```python
from build123d import *

# Parameters (mm, degrees)
SKETCH_2_R          = 0.8
CUT_EXTRUDE_1_DEPTH = 10
CHAMFER_1_SIZE      = 0.5


with BuildPart() as part:
    # Эскиз1 → Повернуть1 (revolve)
    with BuildSketch(Plane(origin=(0, 0, 0), x_dir=(0, 0, -1), z_dir=(1, 0, 0))):
        Polygon((0, 2.5), (0, 5), (2, 5), (2, 3), (38, 3), (38, 2.5), (42, 2.5), (42, 2.95), (43, 2.95), (43, 0), (0, 0), (-5, 0), (-5, 2.95), (-4, 2.95), (-4, 2.5), align=None)
    revolve(axis=Axis((0, 0, 0), (0, 0, -1)))

    # Эскиз2 → Вытянуть1 (cut, symmetric)
    with BuildSketch(Plane(origin=(0, 0, 0), x_dir=(0, 0, -1), z_dir=(1, 0, 0))):
        with Locations((36, 0)):
            Circle(SKETCH_2_R)
    extrude(amount=CUT_EXTRUDE_1_DEPTH, both=True, mode=Mode.SUBTRACT)

    # Фаска1
    chamfer_1_edges = [part.edges().sort_by_distance(p)[0] for p in [
        (0, -2.95, -43),
        (0, -2.95, 5),
    ]]
    chamfer(chamfer_1_edges, length=CHAMFER_1_SIZE)


solid = part.part
```
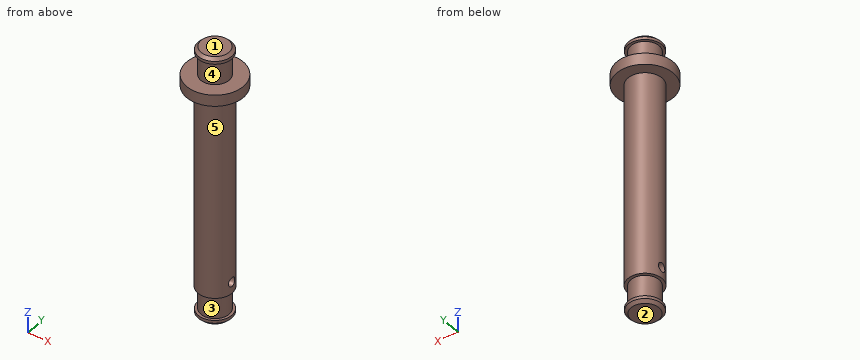
The listing builds one solid part. Answer for the finished solid, in the listing's coordinates (mm). Face numbers are marked on the shaded views. A direction names the side the tool comes from. Coordinates: 2 decimals unless noted, no trailing zeros. Write each loop counter-clockwise with the first axis right and the second up, starting at its lowest first coordinate (ties: lowest second). Pieces come first, ordered by that corner, then holes. Notation, with made-up numbers: (87, 69) - (139, 69) arc R17 cw to (139, 77) - close; hole circle Ø11 at (-22.75, 65.5). An arc over 180 degrees is marked (long way). Return JSON: item names as keys, results as strings. Group by question number.
1. Straight lines are drawn through the part: L1, parallel to Z at x = 0, y = 0; L2, parallel to Z at x = 2.25, y = 1.75; L3, parallel to X at y = -0.25, z = -27. For each, find the intervals that lie inside material, in ascending order.
2. A cutting plane is placed at D-D, the plane x = 4.5. Determine the outline of the cut face in (y, z).
3. Given pin 1 (1.5 mm diameter, centred on y = 2.5, z = -1.5, fed in from -X); pin 2 (1.5 mm diameter, centred on y = 2.5, z = -25.5, fed in from +X); pin 3 (2.5 mm diameter, centred on y = 0, z = -36, fed in from -X); pin 4 (4 mm diameter, centred on x = -1.5, y = -2, fed in from -Z), each flat-ended and moving along its own axis, determine where each tip first touches the part or whether it passes through.
4. A cutting plane is placed at C-C, the plane z = -36. Determine the outline of the cut face in (x, y).
5. Which of the six approach directions +Z, -Z, +X, -X, +Y, -Y give full straight-line access (tool end or side, diameter ignored) to the marked faces 4 and 5?
6. Determine the mould class of the marked faces 1, 2 and 3 for opening direction Z: released by +Z, released by -Z, zero draft, split by the parting line, or undercut.
Ans:
{
 "1": {"L1": "-43 to -36.8, -35.2 to 5", "L2": "-42.6 to -42, -38 to 0, 4 to 4.6", "L3": "-2.99 to 2.99"},
 "2": {"outline": "(-2.18, -2) - (2.18, -2) - (2.18, 0) - (-2.18, 0) - close"},
 "3": {"pin 1": "x = -4.68", "pin 2": "x = 2.44", "pin 3": "x = -3", "pin 4": "z = -43"},
 "4": {"outline": "(-2.89, -0.8) arc R3 ccw to (2.89, -0.8) - close; (-2.89, 0.8) - (2.89, 0.8) arc R3 ccw to start"},
 "5": {"face 4": "none", "face 5": "-Z"},
 "6": {"face 1": "released by +Z", "face 2": "released by -Z", "face 3": "undercut"}
}
